from build123d import *

# Parameters (mm, degrees)
SKETCH1_R          = 38.928100528
SKETCH1_R_2        = 25.022354689
EXTRUDE1_DEPTH     = 3
SKETCH2_W          = 13.898513907
SKETCH2_H          = 1.587850138
EXTRUDE2_DEPTH     = 2
CIRPATTERN1_COUNT  = 24
LPATTERN1_COUNT    = 2
LPATTERN1_PITCH    = 5
EXTRUDE3_START     = -3
SKETCH3_R          = 25.022354689
SKETCH3_R_2        = 22.022354689
EXTRUDE3_DEPTH     = 14
EXTRUDE4_START     = -4
SKETCH4_R          = 22.022354689
SKETCH4_R_2        = 7.022354689
EXTRUDE4_DEPTH     = 4
SKETCH5_R          = 2.374357642
CUT_EXTRUDE1_DEPTH = 4
CIRPATTERN2_COUNT  = 4


with BuildPart() as part:
    # Sketch1 → Extrude1 (new body)
    with BuildSketch(Plane.XY):
        Circle(SKETCH1_R)
        Circle(SKETCH1_R_2, mode=Mode.SUBTRACT)
    extrude1 = extrude(amount=EXTRUDE1_DEPTH)

    # Sketch2 → Extrude2 (add)
    with BuildSketch(Plane.XY.offset(3)):
        with Locations((31.965311014, 0)):
            Rectangle(SKETCH2_W, SKETCH2_H)
    extrude2 = extrude(amount=EXTRUDE2_DEPTH)

    # CirPattern1: Extrude2 ×24 about axis
    cirpattern1_axis = Axis((0, 0, 0), (0, 0, 1))
    for i in range(1, CIRPATTERN1_COUNT):
        add(extrude2.rotate(cirpattern1_axis, i * 360 / CIRPATTERN1_COUNT))

    # LPattern1: Extrude1 ×2
    with Locations(*[(0, 0, i * LPATTERN1_PITCH) for i in range(1, LPATTERN1_COUNT)]):
        add(extrude1)

    # Sketch3 → Extrude3 (add)
    with BuildSketch(Plane.XY.offset(8).offset(EXTRUDE3_START)):
        with Locations(Location((0, 0, 0), (0, 0, 181.285803534))):
            Circle(SKETCH3_R)
        Circle(SKETCH3_R_2, mode=Mode.SUBTRACT)
    extrude(amount=EXTRUDE3_DEPTH)

    # Sketch4 → Extrude4 (add)
    with BuildSketch(Plane.XY.offset(19).offset(EXTRUDE4_START)):
        Circle(SKETCH4_R)
        Circle(SKETCH4_R_2, mode=Mode.SUBTRACT)
    extrude(amount=EXTRUDE4_DEPTH)

    # Sketch5 → Cut-Extrude1 (cut)
    with BuildSketch(Plane.XY.offset(19)):
        with Locations((0, 16.045543099)):
            Circle(SKETCH5_R)
    cut_extrude1 = extrude(amount=-CUT_EXTRUDE1_DEPTH, mode=Mode.SUBTRACT)

    # CirPattern2: Cut-Extrude1 ×4 about axis
    cirpattern2_axis = Axis((0, 0, 0), (0, 0, 1))
    for i in range(1, CIRPATTERN2_COUNT):
        add(cut_extrude1.rotate(cirpattern2_axis, i * 360 / CIRPATTERN2_COUNT), mode=Mode.SUBTRACT)


solid = part.part
Design review of the part built by this model. Coordinates are the model's own, in mm. A direction names the side the tool comes from. Round coordinates to 2 decimals unless told otherwise and drop trailing zeros. Order: outer loops, then holes, each group sorted by start corner. A loop starts at its lowest first (then second) coordinate and runs counter-clockwise, first axis right, second up.
1) For L1, parallel to Y at x = 0, z = 16.5; L2, parallel to Y at x = 0, z = 10.25; L3, parallel to Z at x = 31.5, y = 4.5, list the stretches that pass through material, from the lowest coordinate up.
The answers:
L1: y = -25.02 to -18.42, -13.67 to -7.02, 7.02 to 13.67, 18.42 to 25.02
L2: y = -25.02 to -22.02, 22.02 to 25.02
L3: z = 0 to 3, 5 to 8
2) Consider section A-A (y = -29). State the section outline as (x, z) points, plus the area to 3 significant figures.
The answers:
outline: (-25.97, 0) - (25.97, 0) - (25.97, 3) - (17.66, 3) - (17.66, 5) - (25.97, 5) - (25.97, 8) - (-25.97, 8) - (-25.97, 5) - (-17.66, 5) - (-17.66, 3) - (-25.97, 3) - close; hole (-15.83, 3) - (-8.59, 3) - (-8.59, 5) - (-15.83, 5) - close; hole (-6.95, 3) - (-0.79, 3) - (-0.79, 5) - (-6.95, 5) - close; hole (0.79, 3) - (6.95, 3) - (6.95, 5) - (0.79, 5) - close; hole (8.59, 3) - (15.83, 3) - (15.83, 5) - (8.59, 5) - close
area: 329 mm2
3) Draft analysis for pull direction Z (two halves, no side actions). For faces 1 (the cylindrical face through (-23.69, -8.05, 13.42)), 2 (the flat face through (28, -15.25, 3.99)), 3 (the flat face through (-27.2, -16.62, 3.99)), state which applies: released by +Z, released by -Z, zero draft, split by the parting line, or undercut.
The answers:
face 1: zero draft
face 2: undercut
face 3: undercut
4) Clearance check with flat-ended pins moving along their axes: pin 1 Ø2 at (x, y) = (9, -0.5) entering from -Z; pin 2 Ø1.7 at (y, z) = (-0.5, 4) entering from -X; pin 3 Ø2 at (x, z) = (35.5, 3.5) entering from -Y; pin 4 Ø4.5 at (x, y) = (0, -16.05) entering from +Z. State where each tip first meets the part, or that it passes through.
The answers:
pin 1: stops at z = 15
pin 2: stops at x = -38.91
pin 3: stops at y = -17.77
pin 4: passes through
5) Machinability: for faces 4 (the flat face through (-30.99, 7.48, 3.99)), 5 (the flat face through (30.99, -7.48, 3.99)), 6 (the flat face through (7.48, 30.99, 3.99)), 7 (the flat face through (16.62, -27.2, 3.99)), which of the approach directions +Z, -Z, +X, -X, +Y, -Y give a long, thin tool a straight path to every point of the face, cutting with its end or side? Answer none if there is none.
The answers:
face 4: -X
face 5: +X
face 6: +Y
face 7: none
6) Consider section B-B (z = 9.25). State the section outline as (x, y) points.
The answers:
outline: circle Ø50.04 at (0, 0); hole circle Ø44.04 at (0, 0)
